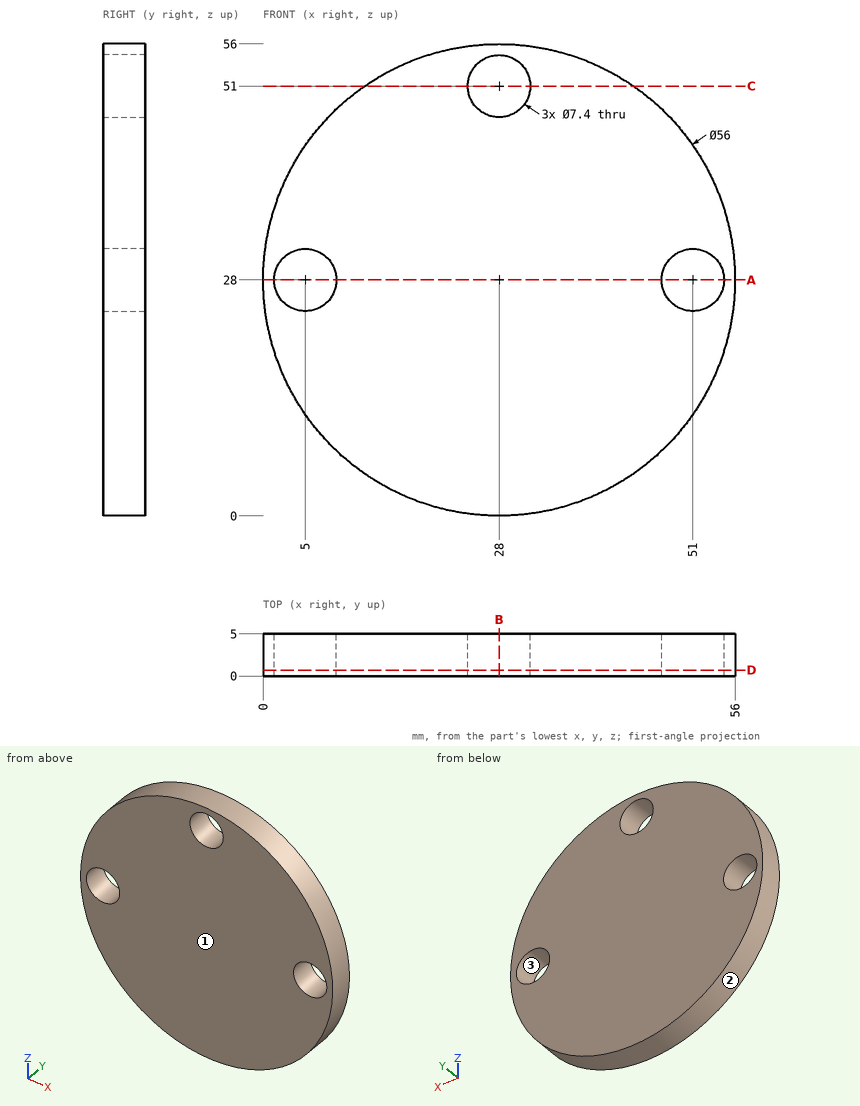
Verification items for this drawing (mm, ordinates from the low corner). Give positions to 0.01 mm unless a question says otherwise; leave off trailing zeros. Loops run counter-clockwise (first coordinate to the right, second up) from the corner with the lowest first, then second, coordinate; pieces in that order, holes last. Notation, with made-up numbers: M 64,79 L 68,79 A28 cw 68,97 Z; hole C -27.5,-0.5 d3. An arc over 180 degrees is marked long. Return JSON: item names as keys, results as strings. Group by question number.
1. Go/stop test with flat-tipped pins: pin 1 (1 mm diameter, centred on x = 13, z = 11, fed in from -Y); pin 2 (1 mm diameter, centred on y = 1.5, z = 24, fed in from -X); pin 3 (2 mm diameter, centred on x = 32, y = 4.5, fed in from -Z). Record where each tip stops, or that it passes through.
2. Cross-section at C-C on z = 51. Record the boundary of the cut face in (x, y).
3. Cross-section at A-A on z = 28. Record the boundary of the cut face in (x, y), plus the area to 3 significant figures.
4. Thickness scan on L1, parallel to X at y = 2.95, z = 28; L2, parallel to Z at x = 3.5, y = 1.2; L3, parallel to Z at x = 3, y = 3.9. Record the ranges inside material, lowest first.
5. Cross-section at D-D on y = 0.7. Record the boundary of the cut face in (x, z).
6. Mould release check, pull along Z, two halves, no side actions. Record for the marked faces 1, 2 and 3: released by +Z, released by -Z, zero draft, split by the parting line, or undercut.
7. Cross-section at B-B on x = 28. Record the boundary of the cut face in (y, z), plus the area to 3 significant figures.
Return value:
{
 "1": {"pin 1": "y = 0", "pin 2": "x = 0.22", "pin 3": "z = 0.16"},
 "2": {"outline": "M 12.03,0 L 24.3,0 L 24.3,5 L 12.03,5 Z; M 31.7,0 L 43.97,0 L 43.97,5 L 31.7,5 Z"},
 "3": {"outline": "M 0,0 L 1.3,0 L 1.3,5 L 0,5 Z; M 8.7,0 L 47.3,0 L 47.3,5 L 8.7,5 Z; M 54.7,0 L 56,0 L 56,5 L 54.7,5 Z", "area": "206 mm^2"},
 "4": {"L1": "0 to 1.3, 8.7 to 47.3, 54.7 to 56", "L2": "14.44 to 24.62, 31.38 to 41.56", "L3": "15.39 to 24.89, 31.11 to 40.61"},
 "5": {"outline": "C 28,28 d56; hole C 5,28 d7.4; hole C 28,51 d7.4; hole C 51,28 d7.4"},
 "6": {"face 1": "zero draft", "face 2": "split by the parting line", "face 3": "undercut"},
 "7": {"outline": "M 0,0 L 5,0 L 5,47.3 L 0,47.3 Z; M 0,54.7 L 5,54.7 L 5,56 L 0,56 Z", "area": "243 mm^2"}
}
